from build123d import *

# Parameters (mm, degrees)
BOSS_EXTRUDE1_DEPTH = 7.95
SHELL1_T            = -1.2
SKETCH2_W           = 1.8
SKETCH2_H           = 5.55
CUT_EXTRUDE1_DEPTH  = 20.473443455
LPATTERN1_COUNT     = 4
LPATTERN1_PITCH     = 3.9


with BuildPart() as part:
    # Sketch1 → Boss-Extrude1 (new body)
    with BuildSketch(Plane.XY):
        Polygon((0, 0), (-15.9, 0), (-15.9, 2.2), (0, 7.95), align=None)
    extrude(amount=-BOSS_EXTRUDE1_DEPTH)

    # Shell1
    shell1_openings = [part.faces().sort_by_distance(p)[0] for p in [
        (-7.95, 0, -3.975),
    ]]
    offset(amount=SHELL1_T, openings=shell1_openings, kind=Kind.INTERSECTION)

    # Sketch2 → Cut-Extrude1 (cut, through all)
    with BuildSketch(Plane.XZ):
        with Locations((-13.8, -3.975)):
            Rectangle(SKETCH2_W, SKETCH2_H)
    cut_extrude1 = extrude(amount=-CUT_EXTRUDE1_DEPTH, mode=Mode.SUBTRACT)

    # LPattern1: Cut-Extrude1 ×4
    with Locations(*[(i * LPATTERN1_PITCH, 0, 0) for i in range(1, LPATTERN1_COUNT)]):
        add(cut_extrude1, mode=Mode.SUBTRACT)


solid = part.part
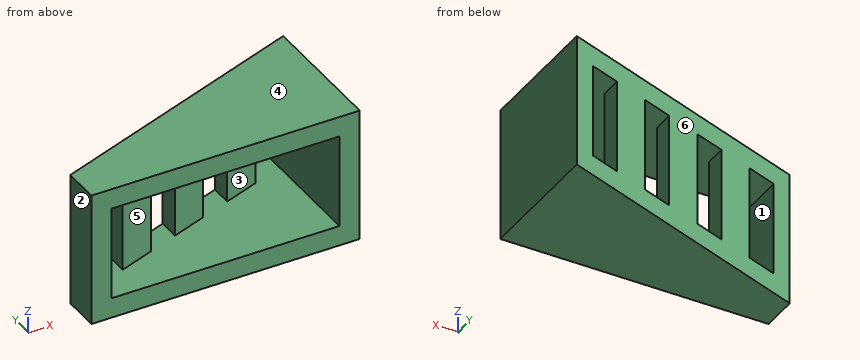
For this review, take the finished solid that the model builds, in its own axes (mm). Face numbers are marked on the shaded views. A direction names the side the tool comes from. Round coordinates to 2 decimals unless told otherwise and drop trailing zeros. Order: outer loops, then holes, each group sorted by start corner. A loop starts at its lowest first (then second) coordinate and runs counter-clockwise, first axis right, second up. Notation, with made-up numbers: M 74,75.25 L 95,75.25 A17 cw 95,92.25 Z; hole C 66,-21 d5. An arc over 180 degrees is marked long. Use a Markdown table: item, result. Add a question column.
Item 1: Add section C-C, the plane x = -11.75. Give the boundary of the cut face in (y, z).
Item 2: Tool access review of the marked faces 1, 2 and 3: name each direction out of +Z, -Z, +X, -X, +Y, -Y from which nothing blocks a thin tool from reaching the whole face with its end or side.
Item 3: To check wall thickness, follow line 1 along Z through (x, y) = (-11.75, 2); line 2 along X through (y, z) = (6, -3); line 3 along X through (y, z) = (7.25, -2.5). State the ranges of each line that lie inside material, in increasing order.
Item 4: Insertion check: pin 1 (3 mm diameter, centred on x = -13.5, z = -3, fed in from +Y). The pin has a flat end and moves straight along its axis. Give the tip position at first contact, or say it passes through.
Item 5: Add section B-B, the plane z = -1.5. Give the boundary of the cut face in (x, y), then the cut area to 3 significant figures.
Item 6: Add section D-D, the plane y = 1.25. Give the boundary of the cut face in (x, z), then the cut area to 3 significant figures.
Item 7: Mouldability with a two-part tool opening along X and no side actions: class the marked faces 4, 5 and 6 as released by +X, released by -X, zero draft, split by the parting line, or undercut.
Item 8: Add section A-A, the plane y = 4.5. Give the boundary of the cut face in (x, z).
Geometry results:
| question | item | result |
|---|---|---|
| 1 | outline | M 0,-7.95 L 3.7,-7.95 L 3.7,0 L 0,0 L 0,-1.2 L 2.42,-1.2 L 2.42,-6.75 L 0,-6.75 Z |
| 2 | face 1 | +Y, -Y |
| 2 | face 2 | +Z, -Z, -X, +Y, -Y |
| 2 | face 3 | -Y |
| 3 | line 1 | z = -7.95 to -6.75, -1.2 to 0 |
| 3 | line 2 | x = -5.1 to -3, -1.2 to 0 |
| 3 | line 3 | x = -1.2 to 0 |
| 4 | pin 1 | stops at y = 3.61 |
| 5 | outline | M -15.9,0 L -14.7,0 L -14.7,2.63 L -15.9,2.2 Z; M -12.9,2.01 L -10.8,2.77 L -10.8,4.04 L -12.9,3.28 Z; M -9,3.42 L -6.9,4.18 L -6.9,5.45 L -9,4.7 Z; M -5.1,4.83 L -3,5.59 L -3,6.87 L -5.1,6.11 Z; M -1.2,0 L 0,0 L 0,7.95 L -1.2,7.52 Z |
| 5 | area | 20.2 mm² |
| 6 | outline | M -15.9,-7.95 L 0,-7.95 L 0,0 L -15.9,0 Z; hole M -14.7,-6.75 L -1.2,-6.75 L -1.2,-1.2 L -14.7,-1.2 Z |
| 6 | area | 51.5 mm² |
| 7 | face 4 | zero draft |
| 7 | face 5 | undercut |
| 7 | face 6 | released by -X |
| 8 | outline | M -9.54,-7.95 L 0,-7.95 L 0,0 L -9.54,0 L -9.54,-1.2 L -9,-1.2 L -9,-6.75 L -9.54,-6.75 Z; hole M -6.9,-6.75 L -1.2,-6.75 L -1.2,-1.2 L -6.9,-1.2 Z |
